The model under review builds one solid part; all positions refer to its coordinate system, in mm. Face numbers are marked on the shaded views. A direction names the side the tool comes from. Round coordinates to 2 decimals unless told otherwise and drop trailing zeros. Order: outer loops, then holes, each group sorted by start corner. A loop starts at its lowest first (then second) coordinate and runs counter-clockwise, first axis right, second up. Notation, with made-up numbers: (27, 52) -> (36, 52) arc R20 cw to (36, 76) -> close; hole circle Ø6 at (38, 7.25). An arc over 180 degrees is marked (long way). Put each result on its own line as item: value. Start each with the question number.
from build123d import *

# Parameters (mm, degrees)
F0_R     = 2.5
F1_DEPTH = 30
F2_R     = 4.5
F3_DEPTH = 4
F4_R     = 2
F6_DEPTH = 4


with BuildPart() as f1:
    # F0 (on Top) → F1 (new body)
    with BuildSketch(Plane.XY):
        Circle(F0_R)
    extrude(amount=F1_DEPTH)

    # F2 (on face) → F3 (join)
    with BuildSketch(Plane.XY.offset(30)):
        Circle(F2_R)
    extrude(amount=F3_DEPTH)

    # F4
    f4_edges = [f1.edges().sort_by_distance(p)[0] for p in [
        (-4.5, 0, 34),
    ]]
    fillet(f4_edges, radius=F4_R)

    # F5 (on face) → F6 (cut)
    with BuildSketch(Plane.XY.offset(34)):
        Polygon((-0.185112, 1.748257), (-1.606591, 0.713817), (-1.421479, -1.03444), (0.185112, -1.748257), (1.606591, -0.713817), (1.421479, 1.03444), align=None)
    extrude(amount=-F6_DEPTH, mode=Mode.SUBTRACT)


solid = f1.part
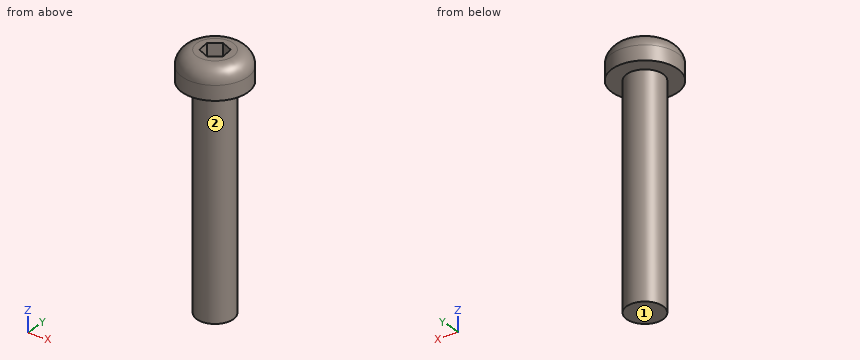
Q1. For the marked faces 1 and 2, list the 3-axis set-ups (+Z, -Z, +X, -X, +Y, -Y) from which the entire face can be reached by the end or side of a thin tool; tool diameter is ignored.
Q2. Take a section at C-C on z = 15.5. Give the boundary of the cut face in (x, y), and give its area (3 significant figures).
Q3. Wall thickness on probe 1 along Z at (x, y) = (1.25, 0.75); probe 2 along Z at (x, y) = (-1.25, -3.25); probe 3 along X at (y, z) = (2.25, 8): over which ranges is each line inside the solid? List them lowest first. Write a range as [from, to].
Q4. Take a section at A-A on z = 31.5. Give the boundary of the cut face in (x, y).
Q5. Clearance check with flat-ended pins moving along their axes: pin 1 Ø1 at (x, z) = (0.5, 25.5) entering from -Y; pin 2 Ø2.5 at (x, y) = (-1.5, 1.5) entering from -Z; pin 3 Ø4 at (y, z) = (1.5, 6) entering from -X; pin 4 Ø5 at (y, z) = (0.5, 15.5) entering from +X. State where each tip first meets the part, or that it passes through.
Q6. Take a section at B-B on y = 0. Give the boundary of the cut face in (x, z).
Calculated:
1. face 1: -Z, +X, -X, +Y, -Y
1. face 2: -Z
2. outline: circle Ø5 at (0, 0)
2. area: 19.6 mm²
3. probe 1: z = [0, 30]
3. probe 2: z = [30, 33.74]
3. probe 3: x = [-1.09, 1.09]
4. outline: circle Ø9 at (0, 0); hole (-1.61, 0.71) -> (-1.42, -1.03) -> (0.19, -1.75) -> (1.61, -0.71) -> (1.42, 1.03) -> (-0.19, 1.75) -> close
5. pin 1: stops at y = -2.5
5. pin 2: stops at z = 0
5. pin 3: stops at x = -2.5
5. pin 4: stops at x = 2.5
6. outline: (-4.5, 30) -> (-2.5, 30) -> (-2.5, 0) -> (2.5, 0) -> (2.5, 30) -> (4.5, 30) -> (4.5, 32) arc R2 ccw to (2.5, 34) -> (1.53, 34) -> (1.53, 30) -> (-1.53, 30) -> (-1.53, 34) -> (-2.5, 34) arc R2 ccw to (-4.5, 32) -> close
